Drawing for the job (mm, zero at the part's lowest x, y, z). A direction names the side the tool comes from. Give positions to 0.01 mm unless a question says otherwise; leave off trailing zeros. Order: outer loops, then holes, each group sorted by start corner. A loop starts at its lowest first (then second) coordinate and runs counter-clockwise, first axis right, second up. Notation, with made-up numbers: (66, -31.75) - (123, -31.75) arc R23 cw to (123, -0.75) - close; hole circle Ø7 at (88.5, 14.25). An arc over 180 degrees is marked (long way). Use a Markdown table: item, result. Add a question column.
(1) Which spindle directions (+Z, -Z, +X, -X, +Y, -Y) get a long thin tool onto all of the face, cutting with end or side? Do the marked faces 1 and 2. Say none if no direction does.
(2) Slice it at A-A (y = 63.5). Write the cut outline in (x, z), then the cut area to 3 significant figures.
(3) Slice it at B-B (z = 17). Write the cut outline in (x, y).
(4) Mould opens along Y. For the marked faces 3, 4, 5 and 6 say: +Y half, -Y half, draft (parallel to the pull), parting line (faces both ways), or undercut.
(5) Wall check: line 1 (Y direction, x = 22.75, z = 16.25); line 2 (X direction, y = 66, z = 15); line 3 (Z direction, x = 18.25, y = 20). Give the ranges that are in metal, low to high.
(6) Slice it at C-C (x = 8.5). Write the cut outline in (y, z), then the cut area to 3 significant figures.
(7) Flat gauge pins, fed straight in: pin 1 (10 mm diameter, centred on x = 7, y = 37, fed in from +Z); pin 2 (4 mm diameter, centred on y = 35, z = 11, fed in from -X); pin 3 (15 mm diameter, centred on y = 25, z = 15.5, fed in from -X). Where does each tip first touch, or does it go through?
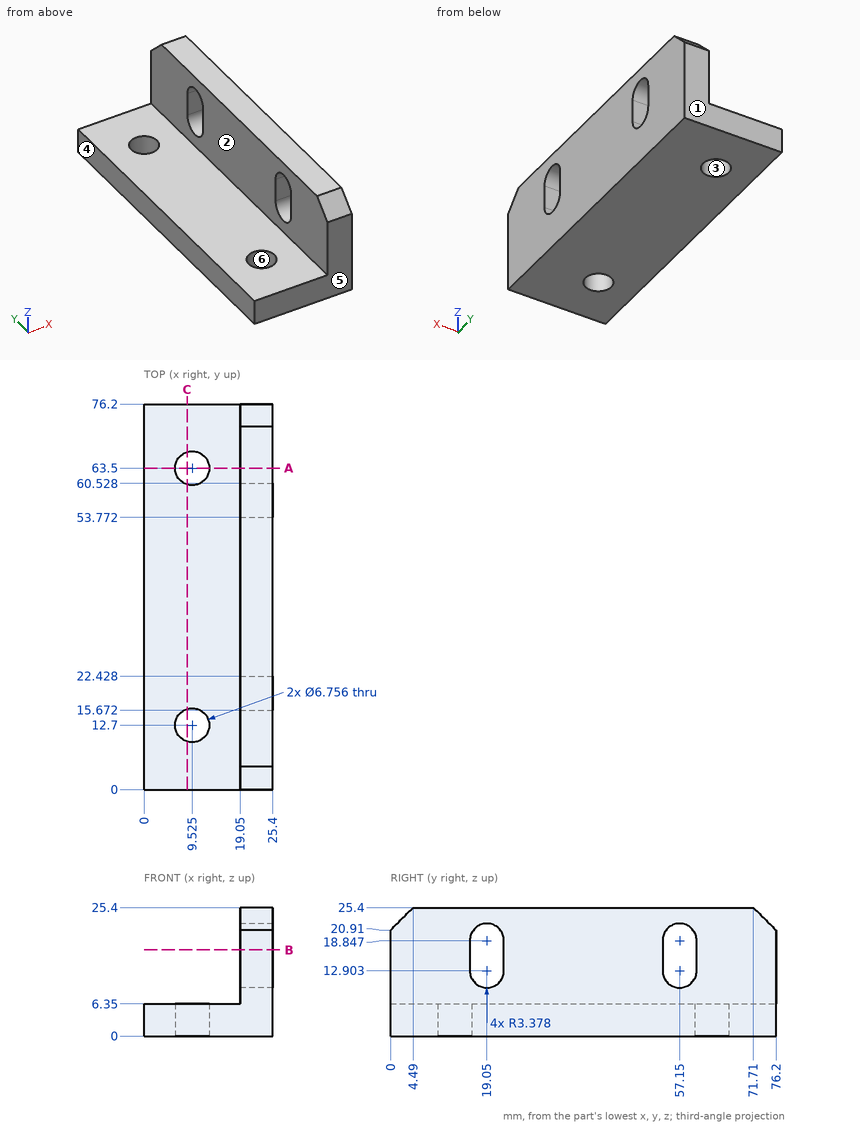
Solution:
| question | item | result |
|---|---|---|
| 1 | face 1 | +Z, -Z, +X, -X, +Y |
| 1 | face 2 | +Z, -X, +Y, -Y |
| 2 | outline | (0, 0) - (6.15, 0) - (6.15, 6.35) - (0, 6.35) - close; (12.9, 0) - (25.4, 0) - (25.4, 25.4) - (19.05, 25.4) - (19.05, 6.35) - (12.9, 6.35) - close |
| 2 | area | 239 mm2 |
| 3 | outline | (19.05, 0) - (25.4, 0) - (25.4, 15.67) - (19.05, 15.67) - close; (19.05, 22.43) - (25.4, 22.43) - (25.4, 53.77) - (19.05, 53.77) - close; (19.05, 60.53) - (25.4, 60.53) - (25.4, 76.2) - (19.05, 76.2) - close |
| 4 | face 3 | undercut |
| 4 | face 4 | draft |
| 4 | face 5 | -Y half |
| 4 | face 6 | undercut |
| 5 | line 1 | 0 to 15.67, 22.43 to 53.77, 60.53 to 76.2 |
| 5 | line 2 | 19.05 to 25.4 |
| 5 | line 3 | 0 to 6.35 |
| 6 | outline | (0, 0) - (9.48, 0) - (9.48, 6.35) - (0, 6.35) - close; (15.92, 0) - (60.28, 0) - (60.28, 6.35) - (15.92, 6.35) - close; (66.72, 0) - (76.2, 0) - (76.2, 6.35) - (66.72, 6.35) - close |
| 6 | area | 402 mm2 |
| 7 | pin 1 | z = 6.35 |
| 7 | pin 2 | x = 19.05 |
| 7 | pin 3 | x = 19.05 |
